Source: CAD feature listing. Evaluate the final solid. Frame: model axes, mm. A direction names the side the tool comes from. Give positions to 0.01 mm unless a question says otherwise; leave off trailing zeros. Loops run counter-clockwise (first coordinate to the right, second up) from the corner with the lowest first, then second, coordinate; pieces in that order, holes last.
from build123d import *

# Parameters (mm, degrees)
F1_DEPTH  = 35
F4_DEPTH  = 29
F5_R      = 6
F6_DEPTH  = 40
F7_W      = 12.2776310586
F7_H      = 2
F8_DEPTH  = 40
F10_DEPTH = 25
F11_R     = 8
F12_R     = 1.625
F12_R_2   = 1.6250003413
F13_DEPTH = 25
F15_W     = 74.6117010713
F15_H     = 42.9684482515
F16_DEPTH = 25
F17_R     = 5


with BuildPart() as f1:
    # F0 (on Top) → F1 (new body)
    with BuildSketch(Plane.XY):
        with BuildLine():
            Line((-48, 0), (0, 0))
            Line((0, 0), (0, 5))
            Line((0, 5), (-48, 5))
            ThreePointArc((-48, 5), (-52.4161984871, 15.4161984871), (-62.8323969742, 11))
            Line((-62.8323969742, 11), (-69.8323969742, 11))
            Line((-69.8323969742, 11), (-69.8323969742, 5))
            Line((-69.8323969742, 5), (-62.8323969742, 5))
            ThreePointArc((-62.8323969742, 5), (-59.8883344421, 1.3667504193), (-55.4161984871, 0))
            Line((-55.4161984871, 0), (-48, 0))
        make_face()
    extrude(amount=F1_DEPTH)

    # F3 (on offset) → F4 (cut)
    with BuildSketch(Plane.XY.offset(35)):
        with BuildLine():
            Line((-56, 0), (-55.9299111582, 0))
            ThreePointArc((-55.9299111582, 0), (-55.9649623523, 0.0030034406), (-56, 0.0061609878))
            Line((-56, 0.0061609878), (-56, 0))
        make_face()
        with BuildLine():
            ThreePointArc((-55.9299111582, 0), (-55.2644431591, -0.0277260244), (-54.59897516, 0))
            Line((-54.59897516, 0), (-55.9299111582, 0))
        make_face()
        with BuildLine():
            Line((-54.59897516, 0), (0, 0))
            Line((0, 0), (0, 5))
            Line((0, 5), (-47.8370891609, 5))
            ThreePointArc((-47.8370891609, 5), (-50.5080325408, 1.5398127025), (-54.59897516, 0))
        make_face()
    extrude(amount=-F4_DEPTH, mode=Mode.SUBTRACT)

    # F5 (on face) → F6 (cut)
    with BuildSketch(Plane.XY.offset(35)):
        with Locations((-55.2644431591, 7.9722739756)):
            Circle(F5_R)
    extrude(amount=-F6_DEPTH, mode=Mode.SUBTRACT)

    # F7 (on offset) → F8 (cut)
    with BuildSketch(Plane.XY.offset(35)):
        with Locations((-64.1601290554, 8)):
            Rectangle(F7_W, F7_H)
    extrude(amount=-F8_DEPTH, mode=Mode.SUBTRACT)

    # F9 (on Front) → F10 (cut)
    with BuildSketch(Plane.XZ):
        Polygon((-74.45092788, 0), (-55.6752420962, 0), (-74.45092788, 18.7756857838), align=None)
    extrude(amount=-F10_DEPTH, mode=Mode.SUBTRACT)

    # F11
    f11_edges = [f1.edges().sort_by_distance(p)[0] for p in [
        (-69.832397, 6, 35),
        (-69.832397, 10, 35),
    ]]
    fillet(f11_edges, radius=F11_R)

    # F12 (on Front) → F13 (cut)
    with BuildSketch(Plane.XZ):
        with Locations((-3.625, 3)):
            Circle(F12_R)
        with Locations((-41.625, 3)):
            Circle(F12_R)
        with Locations((-66.3323969742, 16)):
            Circle(F12_R_2)
        with Locations((-66.3323969742, 26)):
            Circle(F12_R)
    extrude(amount=-F13_DEPTH, mode=Mode.SUBTRACT)

    # F14: F1 across plane


with BuildPart() as f1_1:
    add(f1.part)
    add(f1.part.mirror(Plane.YZ))

    # F15 (on Front) → F16 (cut)
    with BuildSketch(Plane.XZ):
        with Locations((-37.3058505356, 21.4842241257)):
            Rectangle(F15_W, F15_H)
    extrude(amount=-F16_DEPTH, mode=Mode.SUBTRACT)

    # F17
    f17_edges = [f1_1.edges().sort_by_distance(p)[0] for p in [
        (69.832397, 6, 14.157155),
        (69.832397, 10, 14.157155),
    ]]
    fillet(f17_edges, radius=F17_R)


solid = f1_1.part
1) Reachability of faces 1 (the cylindrical face through (49.27, 7.69, 17.74)), 2 (the cylindrical face through (50.458, 1.577, 20.703)), 3 (the flat face through (66, 11, 21)) from +Z, -Z, +X, -X, +Y, -Y: full face, straight path, thin tool, end or side. Return the list, or none.
Checks:
face 1: +Z, -Z
face 2: +Z, -X, -Y
face 3: +Z, -Z, +X, +Y
2) Pull-direction query (Z, two-part tool) for faces 4 (the flat face through (65, 9, 20)), 5 (the cylindrical face through (69.44, 5.99, 14.29)), 6 (the cylindrical face through (5.25, 2.46, 3.07)); classes: released by +Z, released by -Z, zero draft, split by the parting line, or undercut.
Checks:
face 4: zero draft
face 5: released by -Z
face 6: undercut
3) Cut plane D-D (z = 3). Return loops of the section in (x, y), and give its area (3 significant figures).
Checks:
outline: (0, 0) - (2, 0) - (2, 5) - (0, 5) - close; (5.25, 0) - (40, 0) - (40, 5) - (5.25, 5) - close; (43.25, 0) - (55.42, 0) arc R8 ccw to (58.68, 0.69) - (58.68, 3.04) arc R6 cw (long way) to (58.68, 12.91) - (58.68, 15.31) arc R8 ccw to (48, 5) - (43.25, 5) - close
area: 274 mm2
4) Cut plane B-B (y = 10.25). Return loops of the section in (x, z) (3 decimals).
Checks:
outline: (47.739, 0) - (49.714, 0) - (49.714, 35) - (47.739, 35) - close; (60.815, 5.14) - (68.368, 12.693) arc R5 ccw to (69.832, 16.228) - (69.832, 27) arc R8 ccw to (61.832, 35) - (60.815, 35) - close; hole circle Ø3.25 at (66.332, 16); hole circle Ø3.25 at (66.332, 26)
5) Contact query for flat-ended pins moving along their axis: P1, Ø4, axis at x = 66.33, z = 16, coming from the -Y side; P2, Ø1, axis at x = 49.5, z = 17, coming from the -Y side; P3, Ø3.5, axis at x = 3.625, z = 3, coming from the -Y side; P4, Ø2, axis at x = 60.5, z = 14.5, coming from the -Y side. Output: stop coordinate, or through.
Checks:
P1: stops at y = 5
P2: stops at y = 1.95
P3: stops at y = 0
P4: stops at y = 1.12
6) Ray query, probe 1 along Z at (x, y) = (44.5, 2); probe 2 along X at (y, z) = (10.5, 20.5); probe 3 along Y at (x, z) = (37, 3.5). Return the intervals inside material, ascending.
Checks:
probe 1: z = 0 to 6
probe 2: x = 47.82 to 49.82, 60.71 to 69.83
probe 3: y = 0 to 5
7) Cut plane A-A (x = 51). Return loops of the section in (y, z).
Checks:
outline: (0, 0) - (3.75, 0) - (3.75, 35) - (1.2, 35) - (1.2, 6) - (0, 6) - close; (12.19, 0) - (14.67, 0) - (14.67, 35) - (12.19, 35) - close
